```python
from build123d import *

# Parameters (mm, degrees)
SKETCH_1_R      = 7
EXTRUDE_1_DEPTH = 10.5
FILLET_1_R      = 1


with BuildPart() as part:
    # Эскиз1 → Вытянуть1 (new body)
    with BuildSketch(Plane(origin=(0, 0, 0), x_dir=(1, 0, 0), z_dir=(0, 1, 0))):
        Polygon((6.523683625, -10.898389115), (12.700123646, 0.200481188), (6.176440021, 11.098870303), (-6.523683625, 10.898389115), (-12.700123646, -0.200481188), (-6.176440021, -11.098870303), align=None)
        with Locations(Location((0, 0, 0), (0, 0, 90))):
            Circle(SKETCH_1_R, mode=Mode.SUBTRACT)
    extrude(amount=EXTRUDE_1_DEPTH)

    # Скругление1
    fillet_1_edges = [part.edges().sort_by_distance(p)[0] for p in [
        (9.438281834, 10.5, -5.649675745),
        (-0.173621802, 10.5, -10.998629709),
        (-9.611903636, 10.5, -5.348953963),
        (-9.438281834, 10.5, 5.649675745),
        (0.173621802, 10.5, 10.998629709),
        (-9.438281834, 0, 5.649675745),
        (-9.611903636, 0, -5.348953963),
        (-0.173621802, 0, -10.998629709),
        (9.611903636, 10.5, 5.348953963),
        (9.438281834, 0, -5.649675745),
        (9.611903636, 0, 5.348953963),
        (0.173621802, 0, 10.998629709),
    ]]
    fillet(fillet_1_edges, radius=FILLET_1_R)


solid = part.part
```
Geometry: final body of the model. Coordinates: model frame, mm. A direction names the side the tool comes from. Round coordinates to 2 decimals unless told otherwise and drop trailing zeros. Loops run counter-clockwise (first coordinate to the right, second up) from the corner with the lowest first, then second, coordinate; pieces in that order, holes last.
Item 1: Section A-A, the plane y = 4.5. Output: boundary loops of the cut face in (x, z), plus the area to 3 significant figures.
Checked values:
outline: (-12.7, 0.2) - (-6.52, -10.9) - (6.18, -11.1) - (12.7, -0.2) - (6.52, 10.9) - (-6.18, 11.1) - close; hole circle Ø14 at (0, 0)
area: 265 mm2
Item 2: Reachability of faces 1 (the cylindrical face through (0.26, 0.3, 10.71)), 2 (the cylindrical face through (-0.26, 0.3, -10.71)), 3 (the cylindrical face through (9.15, 0.3, -5.58)), 4 (the cylindrical face through (0.26, 10.2, 10.71)), 5 (the cylindrical face through (-9.15, 0.3, 5.58)) from +Z, -Z, +X, -X, +Y, -Y: full face, straight path, thin tool, end or side. Return the list, or none.
Checked values:
face 1: +Z, +X, -Y
face 2: -Z, -X, -Y
face 3: -Z, +X, -Y
face 4: +Z, +X, +Y
face 5: +Z, -X, -Y
Item 3: Contact query for flat-ended pins moving along their axis: P1, Ø1, axis at x = 5, y = 2, coming from the -Z side; P2, Ø1.5, axis at y = 6.5, z = -2.5, coming from the +X side; P3, Ø1.5, axis at x = -10, y = 1, coming from the +Z side. Output: stop coordinate, or through.
Checked values:
P1: stops at z = -11.09
P2: stops at x = 11.77
P3: stops at z = 5.96
Item 4: Mould query, pull axis Z, two halves, no side actions, for faces 6 (the flat face through (9.569, 5.19, 5.427)), 7 (the flat face through (2, 10.5, -7)), 8 (the cylindrical face through (6.834, 5.176, 1.517)). Classes: released by +Z, released by -Z, zero draft, split by the parting line, or undercut.
Checked values:
face 6: released by +Z
face 7: zero draft
face 8: undercut
Item 5: Line query: L1, parallel to X at y = 5, z = 0; L2, parallel to Z at x = -0.5, y = 2; L3, parallel to X at y = 9.75, z = -4.5. Output: solid intervals per line, ascending.
Checked values:
L1: x = -12.59 to -7, 7 to 12.59
L2: z = -10.99 to -6.98, 6.98 to 11.01
L3: x = -10.05 to -5.36, 5.36 to 10.09
